The listing builds one solid part. Answer for the finished solid, in the listing's coordinates (mm). Face numbers are marked on the shaded views. Coordinates: 2 decimals unless noted, no trailing zeros. Order: outer loops, then holes, each group sorted by start corner. A loop starts at its lowest first (then second) coordinate and runs counter-clockwise, first axis right, second up.
from build123d import *

# Parameters (mm, degrees)
F1_DEPTH = 1993.9
F2_R     = 12.065
F3_DEPTH = 254
F4_R     = 7.9375
F5_DEPTH = 6.35


with BuildPart() as f1:
    # F0 (on Front) → F1 (new body)
    with BuildSketch(Plane.XZ):
        with BuildLine():
            Line((-101.273338, 0), (0, 0))
            Line((0, 0), (0, 139.7))
            Line((0, 139.7), (146.05, 139.7))
            Line((146.05, 139.7), (146.05, 73.025))
            Line((146.05, 73.025), (152.4, 73.025))
            Line((152.4, 73.025), (152.4, 89.535))
            ThreePointArc((152.4, 89.535), (194.283381, 119.493668), (224.242049, 161.377049))
            Line((224.242049, 161.377049), (224.242049, 508))
            Line((224.242049, 508), (-101.273338, 508))
            Line((-101.273338, 508), (-101.273338, 0))
        make_face()
    extrude(amount=F1_DEPTH)

    # F2 (on face) → F3 (cut)
    with BuildSketch(Plane.YZ):
        with Locations((-1536.7, 88.9)):
            Circle(F2_R)
        with Locations((-508, 76.2)):
            Circle(F2_R)
    extrude(amount=-F3_DEPTH, mode=Mode.SUBTRACT)

    # F4 (on face) → F5 (join)
    with BuildSketch(Plane(origin=(0, 0, 0), x_dir=(1, 0, 0), z_dir=(0, 0, -1))):
        Polygon((-101.273338, 1460.5), (-101.273338, 1625.6), (-266.373338, 1625.6), (-151.579931, 1460.5), align=None)
        with Locations((-202.873338, 1590.675)):
            Circle(F4_R, mode=Mode.SUBTRACT)
    extrude(amount=-F5_DEPTH)


solid = f1.part
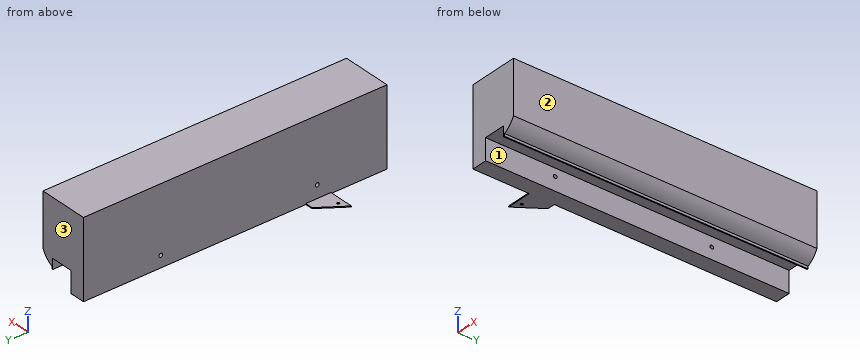
1) Determine the mould class of the marked faces 1, 2 and 3 for opening direction X: released by +X, released by -X, zero draft, split by the parting line, or undercut.
2) Section A-A (y = -821) is taken. Give the vertices of the cut face in (x, z) (3 decimals), then the cut area to 3 significant figures.
3) Section B-B (z = 322.5) is taken. Give the vertices of the cut face in (x, y), then the cut area to 3 significant figures.
4) Each of these flat-tipped pins is pushed along its axis until it touches: P1, Ø1.5, axis at y = -357.5, z = 434.5, coming from the -X side; P2, Ø3, axis at x = -126, z = 4, coming from the +Y side; P3, Ø8, axis at x = 19, y = -1576, coming from the -Z side. Where does it stop, or does it pass through?
5) Consider L1, parallel to Z at x = -22, y = -508 (3 decimals); L2, parallel to Y at x = -46, z = 76; L3, parallel to X at y = -760.5, z = 287. Determine where each line is inside the solid, lowest interval first.
6) Section C-C (x = -172) is taken. Give the vertices of the cut face in (y, z), then the cut area to 3 significant figures.
Filled sheet:
1. face 1: undercut
1. face 2: released by +X
1. face 3: zero draft
2. outline: (-101.273, 0) - (0, 0) - (0, 139.7) - (146.05, 139.7) - (146.05, 73.025) - (152.4, 73.025) - (152.4, 89.535) arc R157.242 ccw to (224.242, 161.377) - (224.242, 508) - (-101.273, 508) - close
2. area: 136,000 mm2
3. outline: (-101.27, -1993.9) - (224.24, -1993.9) - (224.24, 0) - (-101.27, 0) - close
3. area: 649,000 mm2
4. P1: stops at x = -101.27
4. P2: stops at y = -1460.5
4. P3: stops at z = 139.7
5. L1: z = 0 to 64.135, 88.265 to 508
5. L2: y = -1993.9 to -520.06, -495.94 to 0
5. L3: x = -101.27 to 224.24
6. outline: (-1625.6, 0) - (-1489.87, 0) - (-1489.87, 6.35) - (-1625.6, 6.35) - close
6. area: 862 mm2
